Drawing for the job (mm, zero at the part's lowest x, y, z). A direction names the side the tool comes from. Round coordinates to 2 decimals unless told otherwise and drop trailing zeros. Order: outer loops, then holes, each group sorted by start corner. A loop starts at its lowest first (then second) coordinate and runs counter-clockwise, first axis right, second up. Notation, with made-up numbers: M 73,-34.75 L 103,-34.75 A12 cw 103,-17.75 Z; hole C 69,-9.75 d11. An arc over 180 degrees is marked long. One line per item, written item: value. Start each with the question number.
Item 1: Pin check, flat tips, straight feed: pin 1 (8 mm diameter, centred on x = 9, y = 7.5, fed in from +Z); pin 2 (7 mm diameter, centred on x = 38.5, y = 12.5, fed in from +Z). Stop position of each tip, or through.
Item 2: Band-saw the part on A-A, the plane x = 22. Write the cut outline in (y, z).
Item 3: Band-saw the part on C-C, the plane y = 9.87. Write the cut outline in (x, z), then the cut area to 3 significant figures.
Item 4: Band-saw the part on D-D, the plane x = 53.25. Write the cut outline in (y, z).
Item 5: Tool access for the marked faces 1, 2, 3 and 4: list every direction of +Z, -Z, +X, -X, +Y, -Y with a clear straight run to the whole face (end or side of a thin tool).
Item 6: Probe L1, parallel to Y at x = 53.25, z = 32.4; L2, parallel to Z at x = 29, y = 0.6; L3, parallel to Y at x = 45, z = 9. List the from-to ranges inside material, lowest first.
Item 7: Band-saw the part on B-B, the plane z = 5.13. Write the cut outline in (x, y).
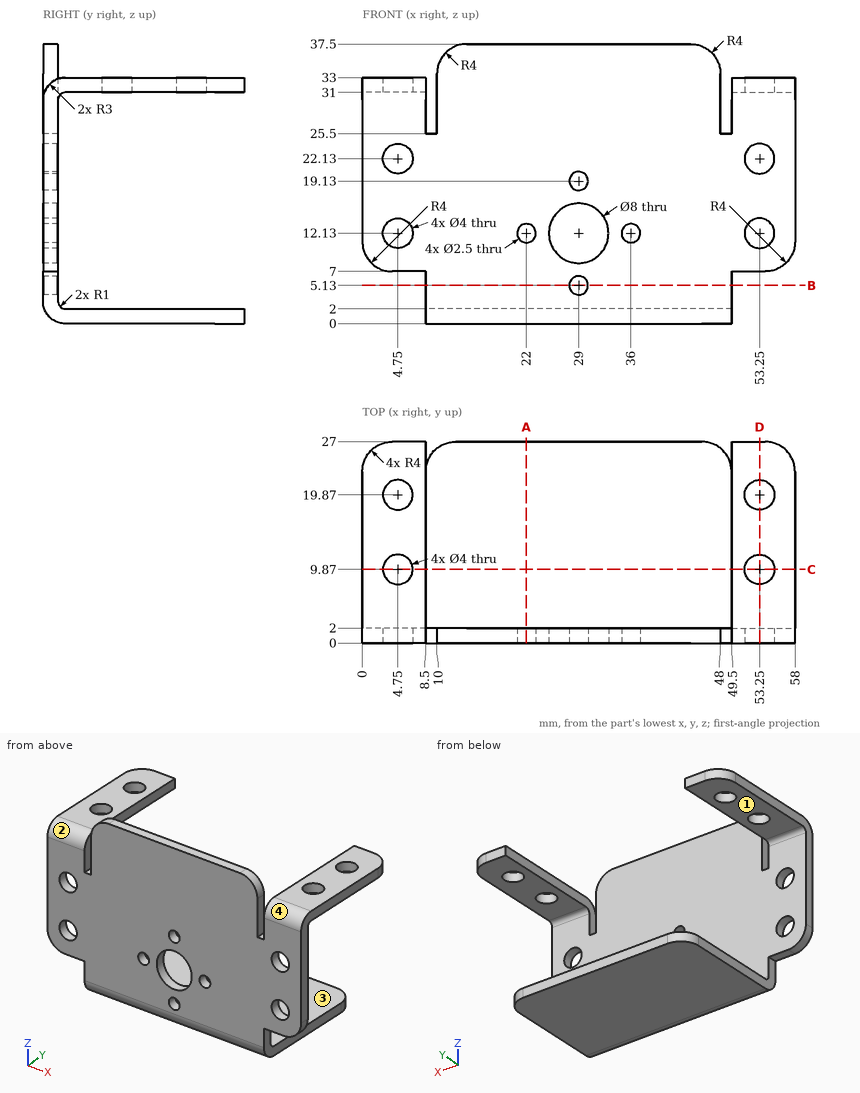
Output:
1. pin 1: stops at z = 33
1. pin 2: stops at z = 2
2. outline: M 0,3 A3 ccw 3,0 L 27,0 L 27,2 L 3,2 A1 cw 2,3 L 2,10.88 L 0,10.88 Z; M 0,13.38 L 2,13.38 L 2,37.5 L 0,37.5 Z
3. outline: M 0,31 L 2.75,31 L 2.75,33 L 0,33 Z; M 6.75,31 L 8.5,31 L 8.5,33 L 6.75,33 Z; M 8.5,0 L 49.5,0 L 49.5,2 L 8.5,2 Z; M 49.5,31 L 51.25,31 L 51.25,33 L 49.5,33 Z; M 55.25,31 L 58,31 L 58,33 L 55.25,33 Z
3. area: 100 mm²
4. outline: M 0,7 L 2,7 L 2,10.13 L 0,10.13 Z; M 0,14.13 L 2,14.13 L 2,20.13 L 0,20.13 Z; M 0,24.13 L 2,24.13 L 2,30 A1 cw 3,31 L 7.87,31 L 7.87,33 L 3,33 A3 ccw 0,30 Z; M 11.87,31 L 17.87,31 L 17.87,33 L 11.87,33 Z; M 21.87,31 L 27,31 L 27,33 L 21.87,33 Z
5. face 1: -Z, +X, -X, +Y
5. face 2: +Z, -X, -Y
5. face 3: +Z, +X, -X, +Y
5. face 4: +Z, +X, -Y
6. L1: y = 1.2 to 7.87, 11.87 to 17.87, 21.87 to 27
6. L2: z = 1.2 to 3.88, 6.38 to 8.13, 16.13 to 17.88, 20.38 to 37.5
6. L3: y = 0 to 2
7. outline: M 8.5,0 L 27.75,0 L 27.75,2 L 8.5,2 Z; M 30.25,0 L 49.5,0 L 49.5,2 L 30.25,2 Z
